```python
from build123d import *

# Parameters (mm, degrees)
SKETCH1_R           = 20.75
SKETCH1_R_2         = 16.5
BOSS_EXTRUDE1_DEPTH = 40
SKETCH2_W           = 10
SKETCH2_H           = 20
CUT_EXTRUDE1_DEPTH  = 20
CIRPATTERN1_COUNT   = 6
FILLET1_R           = 2


with BuildPart() as part:
    # Sketch1 → Boss-Extrude1 (new body)
    with BuildSketch(Plane(origin=(0, 0, 0), x_dir=(1, 0, 0), z_dir=(0, 1, 0))):
        with Locations(Location((0, 0, 0), (0, 0, 270))):
            Circle(SKETCH1_R)
        with Locations(Location((0, 0, 0), (0, 0, 270))):
            Circle(SKETCH1_R_2, mode=Mode.SUBTRACT)
    extrude(amount=BOSS_EXTRUDE1_DEPTH)

    # Sketch2 → Cut-Extrude1 (cut)
    with BuildSketch(Plane.XY.offset(20.75)):
        with BuildLine():
            Line((-5, 10), (5, 10))
            ThreePointArc((5, 10), (0, 5), (-5, 10))
        make_face()
        with Locations((0, 20)):
            Rectangle(SKETCH2_W, SKETCH2_H)
        with BuildLine():
            ThreePointArc((-5, 30), (0, 35), (5, 30))
            Line((5, 30), (-5, 30))
        make_face()
    cut_extrude1 = extrude(amount=-CUT_EXTRUDE1_DEPTH, mode=Mode.SUBTRACT)

    # CirPattern1: Cut-Extrude1 ×6 about axis
    cirpattern1_axis = Axis((0, 0, 0), (0, 1, 0))
    for i in range(1, CIRPATTERN1_COUNT):
        add(cut_extrude1.rotate(cirpattern1_axis, i * 360 / CIRPATTERN1_COUNT), mode=Mode.SUBTRACT)

    # Fillet1
    fillet1_edges = [part.edges().sort_by_distance(p)[0] for p in [
        (0, 40, -20.75),
        (0, 0, -16.5),
        (0, 40, -16.5),
    ]]
    fillet(fillet1_edges, radius=FILLET1_R)


solid = part.part
```
The listing builds one solid part. Answer for the finished solid, in the listing's coordinates (mm). A direction names the side the tool comes from. Coordinates: 2 decimals unless noted, no trailing zeros. Write each loop counter-clockwise with the first axis right and the second up, starting at its lowest first coordinate (ties: lowest second). Pieces come first, ordered by that corner, then holes. Notation, with made-up numbers: (27.5, 80) - (36.5, 80) arc R17 cw to (36.5, 101) - close; hole circle Ø3 at (-21, 10). An arc over 180 degrees is marked (long way). Return JSON: item names as keys, results as strings. Group by question number.
1. Determine the mould class of faces 1 (the flat face through (-5, 20, -18)), 2 (the flat face through (13.056, 19.86, 13.311)), 3 (the flat face through (18.056, 19.86, -4.651)) for opening direction Z: released by +Z, released by -Z, zero draft, split by the parting line, or undercut.
2. Given pin 1 (6 mm diameter, centred on x = -13, z = 9, fed in from -Y); pin 2 (1.3 mm diameter, centred on y = 24, z = 18.5, fed in from +X); pin 3 (1.5 mm diameter, centred on y = 18.5, z = 14.5, fed in from +X); pin 4 (1.3 mm diameter, centred on y = 22, z = -17.5, fed in from -X), each flat-ended and moving along its own axis, determine where each tip first touches the part or whether it passes through.
3. Which of the six approach directions +Z, -Z, +X, -X, +Y, -Y give full straight-line access (tool end or side, diameter ignored) to faces 4 (the flat face through (-18.056, 19.86, -4.651)), 5 (the flat face through (-5, 20, 18)), 6 (the cylindrical face through (15.88, 35, -9.04)), 7 (the flat face through (-13.056, 19.86, -13.311))?
4. A cutting plane is placed at D-D, the plane y = 32. Determine the outline of the cut face in (x, z), plus the area to 3 significant figures.
5. Straight lines are drawn through the part: L1, parallel to X at y = 17, z = 0; L2, parallel to Z at x = 10, y = 28.5; L3, parallel to Z at x = 11.5, y = 26. For each, find the intervals that lie inside material, in ascending order.
6. A cutting plane is placed at C-C, the plane x = 0. Determine the outline of the cut face in (y, z).
7. A cutting plane is placed at B-B, the plane z = 0. Determine the outline of the cut face in (x, y), plus the area to 3 significant figures.
8. A cutting plane is placed at A-A, the plane y = 26. Determine the outline of the cut face in (x, z).
Ans:
{
 "1": {"face 1": "zero draft", "face 2": "undercut", "face 3": "released by -Z"},
 "2": {"pin 1": "y = 0", "pin 2": "x = 10.58", "pin 3": "x = 14.94", "pin 4": "x = -12.11"},
 "3": {"face 4": "-Z", "face 5": "+Z, -Z", "face 6": "none", "face 7": "-X"},
 "4": {"outline": "(-19.82, -6.15) - (-16.02, -3.96) arc R16.5 cw to (-16.02, 3.96) - (-19.82, 6.15) arc R20.75 ccw to start; (-15.24, -14.09) arc R20.75 ccw to (-4.58, -20.24) - (-4.58, -15.85) arc R16.5 cw to (-11.44, -11.89) - close; (-15.24, 14.09) - (-11.44, 11.89) arc R16.5 cw to (-4.58, 15.85) - (-4.58, 20.24) arc R20.75 ccw to start; (4.58, -20.24) arc R20.75 ccw to (15.24, -14.09) - (11.44, -11.89) arc R16.5 cw to (4.58, -15.85) - close; (4.58, 15.85) arc R16.5 cw to (11.44, 11.89) - (15.24, 14.09) arc R20.75 ccw to (4.58, 20.24) - close; (16.02, -3.96) - (19.82, -6.15) arc R20.75 ccw to (19.82, 6.15) - (16.02, 3.96) arc R16.5 cw to start", "area": "261 mm²"},
 "5": {"L1": "-20.75 to -16.5, 16.5 to 20.75", "L2": "-18.18 to -13.12, 13.12 to 18.18", "L3": "-17.27 to -12.41, 12.41 to 17.27"},
 "6": {"outline": "(0, -20.75) - (5, -20.75) - (5, -16.5) - (2, -16.5) arc R2 ccw to (0, -18.5) - close; (0, 18.5) arc R2 ccw to (2, 16.5) - (5, 16.5) - (5, 20.75) - (0, 20.75) - close; (35, -20.75) - (38, -20.75) arc R2 ccw to (40, -18.75) - (40, -18.5) arc R2 ccw to (38, -16.5) - (35, -16.5) - close; (35, 16.5) - (38, 16.5) arc R2 ccw to (40, 18.5) - (40, 18.75) arc R2 ccw to (38, 20.75) - (35, 20.75) - close"},
 "7": {"outline": "(-20.75, 0) - (-18.5, 0) arc R2 ccw to (-16.5, 2) - (-16.5, 38) arc R2 ccw to (-18.5, 40) - (-18.75, 40) arc R2 ccw to (-20.75, 38) - close; (16.5, 2) arc R2 ccw to (18.5, 0) - (20.75, 0) - (20.75, 38) arc R2 ccw to (18.75, 40) - (18.5, 40) arc R2 ccw to (16.5, 38) - close", "area": "335 mm²"},
 "8": {"outline": "(-19.94, -5.74) - (-16.12, -3.53) arc R16.5 cw to (-16.12, 3.53) - (-19.94, 5.74) arc R20.75 ccw to start; (-14.94, -14.4) arc R20.75 ccw to (-5, -20.14) - (-5, -15.72) arc R16.5 cw to (-11.12, -12.19) - close; (-14.94, 14.4) - (-11.12, 12.19) arc R16.5 cw to (-5, 15.72) - (-5, 20.14) arc R20.75 ccw to start; (5, -20.14) arc R20.75 ccw to (14.94, -14.4) - (11.12, -12.19) arc R16.5 cw to (5, -15.72) - close; (5, 15.72) arc R16.5 cw to (11.12, 12.19) - (14.94, 14.4) arc R20.75 ccw to (5, 20.14) - close; (16.12, -3.53) - (19.94, -5.74) arc R20.75 ccw to (19.94, 5.74) - (16.12, 3.53) arc R16.5 cw to start"}
}
